Design review of the part built by this model. Coordinates are the model's own, in mm. A direction names the side the tool comes from. Round coordinates to 2 decimals unless told otherwise and drop trailing zeros. Write each loop counter-clockwise with the first axis right and the second up, starting at its lowest first coordinate (ties: lowest second). Pieces come first, ordered by that corner, then holes.
from build123d import *

# Parameters (mm, degrees)
SKETCH1_R          = 4.191
BASE_EXTRUDE_DEPTH = 7.62
SCALE1_SCALE       = 5.55


with BuildPart() as part:
    # Sketch1 → Base-Extrude (new body)
    with BuildSketch(Plane(origin=(0, 0, 0), x_dir=(1, 0, 0), z_dir=(0, 1, 0))):
        Circle(SKETCH1_R)
    extrude(amount=BASE_EXTRUDE_DEPTH)

    # Sketch2 → Boss-Revolve1 (revolve)
    with BuildSketch(Plane.XY):
        with BuildLine():
            Line((0, 22.987), (0, 6.477))
            ThreePointArc((0, 6.477), (8.255, 14.732), (0, 22.987))
        make_face()
    revolve(axis=Axis((0, 0, 0), (0, 1, 0)))


with BuildPart() as part_1:
    # Scale1: scaled about (0, 13.146971179, 0)
    add(part.part.scale(SCALE1_SCALE).moved(Location((0, -59.818718864, 0))))


solid = part_1.part
1) For faces 1 (the face through (0, -59.819, 0)), 2 (the face through (22.186, -38.969, -6.987)), list the 3-axis set-ups (+Z, -Z, +X, -X, +Y, -Y) from which the entire face can be reached by the end or side of a thin tool; tool diameter is ignored.
2) Add section C-C on y = -8.5. State the section outline as (x, z) points.
3) Add section B-B on x = 0. State the section outline as (y, z) points, and give its area (3 significant figures).
4) Add section A-A on z = 0. State the section outline as (x, y) points, and give its area (3 significant figures).
5) For P1, Ø1, axis at x = -7, z = -3.5, coming from the +Y side; P2, Ø12, axis at x = 9, y = -21.5, coming from the -Z side; P3, Ø6, axis at y = 24.5, z = -13.5, coming from the -X side, all flat-tipped, find the tip position at first contact; note any pin that passes through.
6) Add section D-D on z = -31.5. State the section outline as (x, y) points, and give its area (3 significant figures).
7) For line 1 along Z through (x, y) = (-3, 16); line 2 along Z through (x, y) = (-32, -6.5); line 3 along Y through (x, z) = (-21.5, -22), list the stretches that pass through material, from the lowest coordinate up.
Computed:
1. face 1: +Z, -Z, +X, -X, -Y
1. face 2: -Y
2. outline: circle Ø68.48 at (0, 0)
3. outline: (-59.82, -23.26) - (-17.53, -23.26) arc R45.82 ccw (long way) to (-17.53, 23.26) - (-59.82, 23.26) - close
3. area: 8,360 mm2
4. outline: (-23.26, -59.82) - (23.26, -59.82) - (23.26, -17.53) arc R45.82 ccw (long way) to (-23.26, -17.53) - close
4. area: 8,360 mm2
5. P1: stops at y = 67.17
5. P2: stops at z = -25.04
5. P3: stops at x = -44.54
6. outline: circle Ø66.54 at (0, 21.94)
6. area: 3,480 mm2
7. line 1: z = -45.33 to 45.33
7. line 2: z = -16.31 to 16.31
7. line 3: y = -12.01 to 55.9
